Source: three-view drawing plus pictorial views. Frame: mm from the lowest corner of the part. Coordinates: 2 decimals unless noted, no trailing zeros. Loops run counter-clockwise (first coordinate to the right, second up) from the corner with the lowest first, then second, coordinate; pieces in that order, holes last. Notation, with made-up numbers: (-12.5, -29.5) - (19.5, -29.5) arc R23 ccw to (19.5, 5.5) - close; hole circle Ø10 at (22.25, 85.25). An arc over 180 degrees is marked (long way). Return JSON: item names as keys, results as strings.
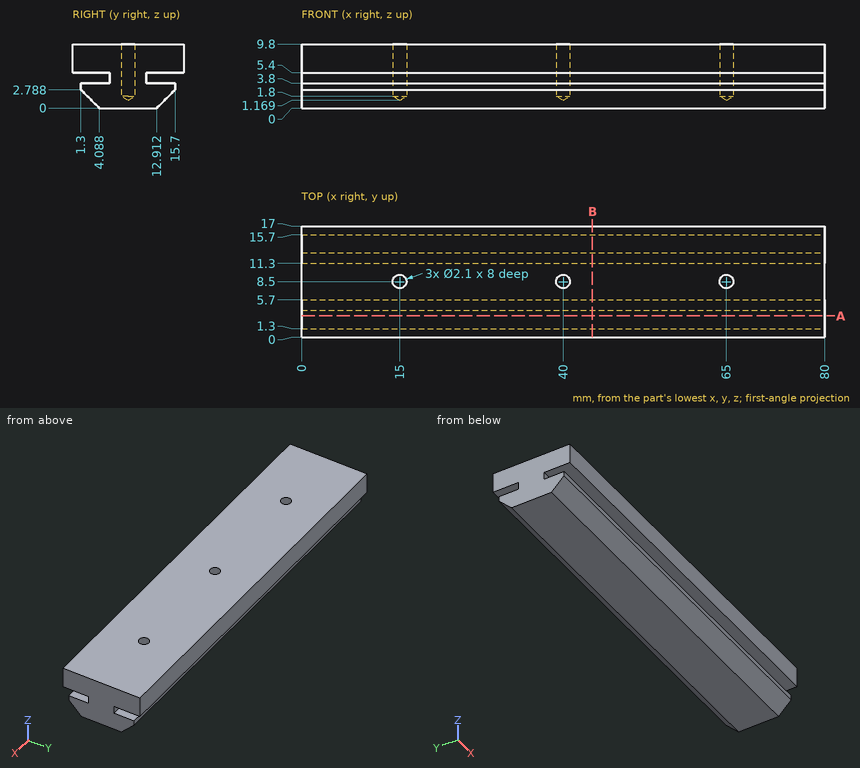
Item 1: First-contact query: pin 1 Ø1.9 at (x, y) = (15, 8.5) entering from +Z; pin 2 Ø1.3 at (x, y) = (65, 8.5) entering from +Z; pin 3 Ø4.5 at (x, y) = (52, 15.5) entering from -Z. Flat tips, straight axial feed; report the tip coordinate or a pass-through.
Worked out:
{"pin 1": "z = 1.74", "pin 2": "z = 1.56", "pin 3": "z = 0.34"}
Item 2: Section query A-A, the plane y = 3.25. Return loops of the section in (x, z).
Worked out:
{"outline": "(0, 0.84) - (80, 0.84) - (80, 3.8) - (0, 3.8) - close; (0, 5.4) - (80, 5.4) - (80, 9.8) - (0, 9.8) - close"}
Item 3: Section query B-B, the plane x = 44.5. Return loops of the section in (y, z), and give its area (3 significant figures).
Worked out:
{"outline": "(0, 5.4) - (5.7, 5.4) - (5.7, 3.8) - (1.3, 3.8) - (1.3, 2.79) - (4.09, 0) - (12.91, 0) - (15.7, 2.79) - (15.7, 3.8) - (11.3, 3.8) - (11.3, 5.4) - (17, 5.4) - (17, 9.8) - (0, 9.8) - close", "area": "131 mm^2"}
Item 4: Ray query, probe 1 along X at (y, z) = (8.5, 5.25); probe 2 along Y at (x, z) = (15, 3.75); probe 3 along Y at (x, z) = (65, 4). Return the intervals inside material, ascending. Write a range as from..to.
Worked out:
{"probe 1": "0..13.95, 16.05..38.95, 41.05..63.95, 66.05..80", "probe 2": "1.3..7.45, 9.55..15.7", "probe 3": "5.7..7.45, 9.55..11.3"}
